Could you check a few things on this model? Use its own coordinates, in mm. A direction names the side the tool comes from. Round coordinates to 2 decimals unless told otherwise and drop trailing zeros. Write each loop counter-clockwise with the first axis right and the second up, starting at its lowest first coordinate (ties: lowest second). Pieces come first, ordered by that corner, then holes.
```python
from build123d import *

# Parameters (mm, degrees)
BOSS_EXTRUDE1_DEPTH     = 15
CUT_EXTRUDE1_DEPTH      = 36.492719011
CUT_EXTRUDE1_DEPTH_BACK = 36.492719011
SKETCH2_R               = 1.5
CHAMFER1_SIZE           = 1.5
FILLET1_R               = 1.5
FILLET2_R               = 1
FILLET3_R               = 1


with BuildPart() as part:
    # Sketch1 → Boss-Extrude1 (new body)
    with BuildSketch(Plane.XY):
        Polygon((0, 0), (11, 0), (11, 3), (9, 3), (9, 1.5), (2, 1.5), (2, 19.5), (11, 19.5), (11, 18), (13, 18), (13, 19.5), (23.094875358, 20.832410877), (25, 22.488510462), (10.837768967, 21), (0, 21), align=None)
    extrude(amount=BOSS_EXTRUDE1_DEPTH)

    # Sketch2 → Cut-Extrude1 (cut, two sides: drawn at the far end of the back side and taken through both)
    with BuildSketch(Plane(origin=(2, 0, 0), x_dir=(0, 0, -1), z_dir=(1, 0, 0)).offset(-CUT_EXTRUDE1_DEPTH_BACK)):
        with Locations(Location((-7.5, 10, 0), (0, 0, 90))):
            Circle(SKETCH2_R)
    extrude(amount=CUT_EXTRUDE1_DEPTH + CUT_EXTRUDE1_DEPTH_BACK, mode=Mode.SUBTRACT)

    # Chamfer1
    chamfer1_edges = [part.edges().sort_by_distance(p)[0] for p in [
        (2, 8.5, 7.5),
    ]]
    chamfer(chamfer1_edges, length=CHAMFER1_SIZE)

    # Fillet1
    # the kernel refuses this fillet: 1.5 mm, written as the material it takes off along each edge
    with BuildSketch(Plane(origin=(9, 3, -3.75), x_dir=(1, 0, 0), z_dir=(0, 0, 1)), Plane(origin=(11, 3, -3.75), x_dir=(0, -1, 0), z_dir=(0, 0, 1)), Plane(origin=(13, 18, -3.75), x_dir=(-1, 0, 0), z_dir=(0, 0, 1)), Plane(origin=(11, 18, -3.75), x_dir=(0, 1, 0), z_dir=(0, 0, 1))) as fillet1_piece_1:
        with BuildLine():
            CenterArc((FILLET1_R, -FILLET1_R), FILLET1_R, 90, 90)
            Line((0, -FILLET1_R), (0, 0))
            Line((0, 0), (FILLET1_R, 0))
        make_face()
    extrude(amount=22.5, mode=Mode.SUBTRACT)

    # Fillet2
    fillet2_edges = [part.edges().sort_by_distance(p)[0] for p in [
        (2, 1.5, 7.5),
        (11, 0, 7.5),
        (10.837768967, 21, 7.5),
        (23.094875358, 20.832410877, 7.5),
        (2, 19.5, 7.5),
    ]]
    fillet(fillet2_edges, radius=FILLET2_R)

    # Fillet3
    fillet3_edges = [part.edges().sort_by_distance(p)[0] for p in [
        (9, 1.5, 7.5),
        (13, 19.5, 7.5),
        (11, 19.5, 7.5),
    ]]
    fillet(fillet3_edges, radius=FILLET3_R)


solid = part.part
```
Q1. Imagine slicing it at C-C, the plane z = 13.75. Write out the boundary of the cut face in (x, y).
Q2. Imagine slicing it at D-D, the plane y = 14. Write out the boundary of the cut face in (x, z).
Q3. Imagine slicing it at A-A, the plane y = 10. Write out the boundary of the cut face in (x, z), then the cut area to 4 significant figures.
Q4. Imagine slicing it at B-B, the plane z = 7.5. Write out the boundary of the cut face in (x, y), then the cut area to 3 significant figures.
Q5. I'm going to push flat-ended pins straight in: pin 1 Ø5 at (y, z) = (10, 7.5) entering from +X; pin 2 Ø10 at (x, y) = (17, 2.5) entering from +Z; pin 3 Ø2.5 at (x, z) = (5, 9) entering from +Y; pin 4 Ø2 at (x, z) = (15.5, 7) entering from +Y. Where does each tip first touch, or does it pass through?
Q6. If I drill on L1, parallel to Y at x = 4.75, z = 11.25; L2, parallel to Y at x = 0.1, z = 7.5; L3, parallel to Z at x = 0.3, y = 10, over which ranges is the centre line in solid material (lowest first)?
Q7. We'd pull the mould along Y, two halves only. Please class faces 1 (the flat face through (5, 21, 7)), 2 (the flat face through (7, 19.5, 7)), 3 (the cylindrical face through (10.763, 19.332, 7.605)), 4 (the cylindrical face through (13.22, 19.39, 7.6)): pulls with the +Y half, pulls with the -Y half, needs draft (parallel to the pull), parting line crosses it, or undercut.
Q8. On a 3-axis mill with a long thin cutter (end or side, diameter ignored), from which of +Z, -Z, +X, -X, +Y, -Y can I reach the whole of each face in a straight line? I mean faces 5 (the cylindrical face through (10.7, 2.4, 7.4)), 6 (the cylindrical face through (9.48, 2.6, 7.4)), 7 (the cylindrical face through (11.47, 18.41, 7.4)). Say none if no direction works.
Results found:
1. outline: (0, 0) - (10, 0) arc R1 ccw to (11, 1) - (11, 1.5) arc R1.5 ccw to (10, 2.91) arc R1.5 ccw to (9.13, 2.1) arc R1 cw to (8.21, 1.5) - (3, 1.5) arc R1 cw to (2, 2.5) - (2, 18.5) arc R1 cw to (3, 19.5) - (10.21, 19.5) arc R1 cw to (11.13, 18.9) arc R1.5 ccw to (12, 18.09) arc R1.5 ccw to (12.9, 18.96) arc R1 cw to (13.7, 19.59) - (22.8, 20.79) arc R1 ccw to (23.32, 21.03) - (25, 22.49) - (10.89, 21.01) arc R1 cw to (10.79, 21) - (0, 21) - close
2. outline: (0, 0) - (2, 0) - (2, 15) - (0, 15) - close
3. outline: (0, 0) - (2, 0) - (2, 4.5) - (0.5, 6) - (0, 6) - close; (0, 9) - (0.5, 9) - (2, 10.5) - (2, 15) - (0, 15) - close
3. area: 21.75 mm2
4. outline: (0, 0) - (10, 0) arc R1 ccw to (11, 1) - (11, 1.5) arc R1.5 ccw to (10, 2.91) arc R1.5 ccw to (9.13, 2.1) arc R1 cw to (8.21, 1.5) - (3, 1.5) arc R1 cw to (2, 2.5) - (2, 7) - (0.5, 8.5) - (0, 8.5) - close; (0, 11.5) - (0.5, 11.5) - (2, 13) - (2, 18.5) arc R1 cw to (3, 19.5) - (10.21, 19.5) arc R1 cw to (11.13, 18.9) arc R1.5 ccw to (12, 18.09) arc R1.5 ccw to (12.9, 18.96) arc R1 cw to (13.7, 19.59) - (22.8, 20.79) arc R1 ccw to (23.32, 21.03) - (25, 22.49) - (10.89, 21.01) arc R1 cw to (10.79, 21) - (0, 21) - close
4. area: 86.1 mm2
5. pin 1: stops at x = 1.5
5. pin 2: passes through
5. pin 3: stops at y = 21
5. pin 4: stops at y = 21.6
6. L1: y = 0 to 1.5, 19.5 to 21
6. L2: y = 0 to 8.5, 11.5 to 21
6. L3: z = 0 to 6, 9 to 15
7. face 1: pulls with the +Y half
7. face 2: undercut
7. face 3: undercut
7. face 4: pulls with the -Y half
8. face 5: +Z, -Z, +X
8. face 6: +Z, -Z
8. face 7: +Z, -Z, -Y
